Check sheet for the modelled part. Datum: model origin and axes. Units: mm. A direction names the side the tool comes from. Round coordinates to 2 decimals unless told otherwise and drop trailing zeros. Write each loop counter-clockwise with the first axis right and the second up, starting at its lowest first coordinate (ties: lowest second). Pieces come first, ordered by that corner, then holes. Notation, with made-up numbers: M 25.5,83.5 L 37.5,83.5 A27 ccw 37.5,100.5 Z; hole C -28,81 d5. An arc over 180 degrees is marked long. One line per item, written item: value.
from build123d import *

# Parameters (mm, degrees)
RESSALTO_EXTRUS_O1_DEPTH = 25
CHANFRO1_SIZE            = 2


with BuildPart() as part:
    # Esboço1 → Ressalto-extrusão1 (new, symmetric)
    with BuildSketch(Plane(origin=(0, 0, 0), x_dir=(0, 0, -1), z_dir=(1, 0, 0))):
        with BuildLine():
            Line((0, 0), (-63, 0))
            Line((-63, 0), (-63, 16.5))
            Line((-63, 16.5), (22, 16.5))
            ThreePointArc((22, 16.5), (39.67766953, 23.82233047), (47, 41.5))
            Line((47, 41.5), (47, 66.5))
            Line((47, 66.5), (50, 66.5))
            Line((50, 66.5), (50, 13.5))
            Line((50, 13.5), (-60, 13.5))
            Line((-60, 13.5), (-60, 3))
            Line((-60, 3), (0, 4))
            Line((0, 4), (0, 3))
            Line((0, 3), (0, 0))
        make_face()
    extrude(amount=RESSALTO_EXTRUS_O1_DEPTH, both=True)

    # Chanfro1
    chanfro1_edges = [part.edges().sort_by_distance(p)[0] for p in [
        (-25, 66.5, -48.5),
        (25, 66.5, -48.5),
    ]]
    chamfer(chanfro1_edges, length=CHANFRO1_SIZE)


solid = part.part
Q1. Sectioned sample at D-D on y = 48.5. Enter the section's corners in (x, z).
Completed:
outline: M -25,-50 L 25,-50 L 25,-47 L -25,-47 Z
Q2. Sectioned sample at C-C on z = 33. Enter the section's corners in (x, y), and give its area (4 significant figures).
Completed:
outline: M -25,0 L 25,0 L 25,3.45 L -25,3.45 Z; M -25,13.5 L 25,13.5 L 25,16.5 L -25,16.5 Z
area: 322.5 mm^2
Q3. Scan lines: line 1 (Z direction, x = 17.5, y = 8); line 2 (Z direction, x = 17.5, y = 52.5); line 3 (Y direction, x = -13.5, z = 48). Record each from-to range of solid material in increasing order. Write a range as [from, to].
Completed:
line 1: [60, 63]
line 2: [-50, -47]
line 3: [0, 3.2], [13.5, 16.5]
Q4. Sectioned sample at B-B on x = 0. Enter the section's corners in (y, z), and give its area (3 significant figures).
Completed:
outline: M 0,0 L 4,0 L 3,60 L 13.5,60 L 13.5,-50 L 66.5,-50 L 66.5,-47 L 41.5,-47 A25 cw 16.5,-22 L 16.5,63 L 0,63 Z
area: 874 mm^2
Q5. Access from +Z, -Z, +X, -X, +Y, -Y to the whole of each face (thin tool, end or side, straight path). Record for faces 4 (the flat face through (0, 54, -47)), 5 (the flat face through (-25, 16, -6)), 6 (the flat face through (0, 2, 0)).
Completed:
face 4: +Z, +X, -X, +Y
face 5: +Z, -Z, -X, +Y, -Y
face 6: -Z, +X, -X, -Y
Q6. Draft check along Y on faces 1 (the flat face through (0, 8, 63)), 2 (the flat face through (0, 16.5, 21)), 3 (the flat face through (0, 13.5, 4)). Enter one of: pulls with the +Y half, pulls with the -Y half, needs draft (parallel to the pull), parting line crosses it, or undercut.
Completed:
face 1: needs draft
face 2: pulls with the +Y half
face 3: undercut
Q7. Sectioned sample at A-A on z = 18. Enter the section's corners in (x, y).
Completed:
outline: M -25,0 L 25,0 L 25,3.7 L -25,3.7 Z; M -25,13.5 L 25,13.5 L 25,16.5 L -25,16.5 Z
Q8. Depth check by flat-ended pin: P1, Ø2, axis at x = -0.5, y = 2, coming from the -Z side; P2, Ø3, axis at x = 4.5, z = -4.5, coming from the +Y side; P3, Ø3, axis at x = 3.5, y = 8, coming from the -Z side. Enter the tip coordinate at first touch or a pass-through.
Completed:
P1: z = 0
P2: y = 16.5
P3: z = 60
